For this review, take the finished solid that the model builds, in its own axes (mm). A direction names the side the tool comes from. Round coordinates to 2 decimals unless told otherwise and drop trailing zeros. Order: outer loops, then holes, each group sorted by start corner. A loop starts at its lowest first (then second) coordinate and runs counter-clockwise, first axis right, second up. Notation, with made-up numbers: (-5.5, 50.25) - (46.5, 50.25) arc R27 cw to (46.5, 68.25) - close; hole circle Ø4 at (80, 50). An arc over 180 degrees is marked (long way). One line per item, written item: value.
```python
from build123d import *

# Parameters (mm, degrees)
F0_W     = 82.709495
F0_H     = 7
F0_R     = 1
F1_DEPTH = 0.8
F2_W     = 12.371881
F2_H     = 7
F3_DEPTH = 60


with BuildPart() as f1:
    # F0 (on Top) → F1 (new body)
    with BuildSketch(Plane.XY):
        with Locations((1.508386, 0.357548)):
            Rectangle(F0_W, F0_H)
        with Locations((-35.321221, 0)):
            Circle(F0_R, mode=Mode.SUBTRACT)
        with Locations((39.078779, 0)):
            Circle(F0_R, mode=Mode.SUBTRACT)
    extrude(amount=F1_DEPTH)

    # F2 (on face) → F3 (join)
    with BuildSketch(Plane.XY.offset(0.8)):
        with Locations((-0.099949, 0.357548)):
            Rectangle(F2_W, F2_H)
    extrude(amount=F3_DEPTH)


solid = f1.part
```
Item 1: For P1, Ø2, axis at y = 0.5, z = 37, coming from the +X side; P2, Ø2.5, axis at x = -35.32, y = 0, coming from the +Z side; P3, Ø3.5, axis at y = 2, z = 33.5, coming from the -X side, all flat-tipped, find the tip position at first contact; note any pin that passes through.
Returned:
P1: x = 6.09
P2: z = 0.8
P3: x = -6.29
Item 2: Take a section at A-A (y = 0). Write out the cut boundary in (x, z).
Returned:
outline: (-39.85, 0) - (-36.32, 0) - (-36.32, 0.8) - (-39.85, 0.8) - close; (-34.32, 0) - (38.08, 0) - (38.08, 0.8) - (6.09, 0.8) - (6.09, 60.8) - (-6.29, 60.8) - (-6.29, 0.8) - (-34.32, 0.8) - close; (40.08, 0) - (42.86, 0) - (42.86, 0.8) - (40.08, 0.8) - close
Item 3: Take a section at C-C (x = 32). Write out the cut boundary in (y, z), plus the area to 3 significant figures.
Returned:
outline: (-3.14, 0) - (3.86, 0) - (3.86, 0.8) - (-3.14, 0.8) - close
area: 5.60 mm^2
Item 4: Machinability: for faces 5 (the flat face through (24, 0, 0.8)), 6 (the flat face through (1, 0, 0)), 7 (the flat face through (-23, 0, 0.8)), which of the approach directions +Z, -Z, +X, -X, +Y, -Y give a long, thin tool a straight path to every point of the face, cutting with its end or side? Answer none if there is none.
Returned:
face 5: +Z, +X, +Y, -Y
face 6: -Z, +X, -X, +Y, -Y
face 7: +Z, -X, +Y, -Y
Item 5: Take a section at B-B (z = 47). Write out the cut boundary in (x, y), plus the area to 3 significant figures.
Returned:
outline: (-6.29, -3.14) - (6.09, -3.14) - (6.09, 3.86) - (-6.29, 3.86) - close
area: 86.6 mm^2
Item 6: The part is to be moulded in two halves that separate along Y. For faces 1 (the flat face through (6.086, 0, 30)), 2 (the flat face through (-2, 3.858, 30)), 3 (the cylindrical face through (-36.058, 0.676, 0.394)), 4 (the cylindrical face through (40.033, 0.3, 0.394)), say which applies: +Y half, -Y half, draft (parallel to the pull), parting line (faces both ways), or undercut.
Returned:
face 1: draft
face 2: +Y half
face 3: undercut
face 4: undercut
Item 7: Wall thickness on line 1 (Z direction, x = 15.5, y = 0); line 2 (X direction, y = -2.5, z = 47): over which ranges is each line inside the solid? List them lowest first.
Returned:
line 1: 0 to 0.8
line 2: -6.29 to 6.09
